```python
from build123d import *

# Parameters (mm, degrees)
EXTRUSION1_DEPTH = 3


with BuildPart() as part:
    # Esquisse1 → Extrusion1 (new body)
    with BuildSketch(Plane.XY):
        with BuildLine():
            Line((150, 232), (-150, 232))
            Line((-150, 232), (-150, 30))
            ThreePointArc((-150, 30), (-135.857864376, 24.142135624), (-130, 10))
            Line((-130, 10), (-130, 0))
            Line((-130, 0), (130, 0))
            Line((130, 0), (130, 10))
            ThreePointArc((130, 10), (135.857864376, 24.142135624), (150, 30))
            Line((150, 30), (150, 232))
        make_face()
        with BuildLine():
            Line((-15, 102), (-15, 132))
            ThreePointArc((-15, 132), (0, 147), (15, 132))
            Line((15, 132), (15, 102))
            ThreePointArc((15, 102), (0, 87), (-15, 102))
        make_face(mode=Mode.SUBTRACT)
        with BuildLine():
            Line((-110, 207), (-110, 217))
            ThreePointArc((-110, 217), (-100, 227), (-90, 217))
            Line((-90, 217), (-90, 207))
            ThreePointArc((-90, 207), (-100, 197), (-110, 207))
        make_face(mode=Mode.SUBTRACT)
    extrude(amount=EXTRUSION1_DEPTH)


solid = part.part
```
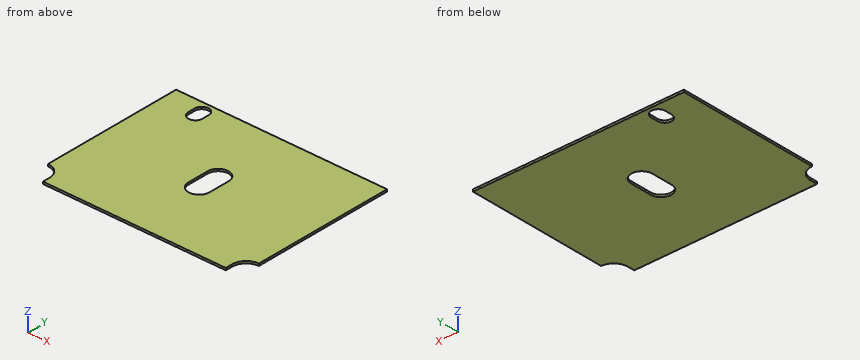
Can you work these out from the model? Positions are in its coordinate system, mm. Give positions to 0.01 mm unless a question says otherwise; leave off trailing zeros. Write each loop counter-clockwise with the first axis right and the second up, starting at its lowest first coordinate (ties: lowest second). Pieces come first, ordered by that corner, then holes. Notation, with made-up numbers: (42.25, 38) -> (96.25, 38) arc R10 ccw to (96.25, 56) -> close; hole circle Ø6 at (-25.5, 35.25). An arc over 180 degrees is marked (long way). One line per item, written item: value.
Q1. Please list where these lines run through material, in increasing order: line 1 (X direction, y = 104, z = 1.7); line 2 (X direction, y = 209, z = 2); line 3 (Y direction, x = 134, z = 0.45). Write a range as [from, to].
Results found:
line 1: x = [-150, -15], [15, 150]
line 2: x = [-150, -110], [-90, 150]
line 3: y = [22, 232]
Q2. Imagine slicing it at B-B on x = -100. Please give me the cut outline in (y, z), and give its area (3 significant figures).
Results found:
outline: (0, 0) -> (197, 0) -> (197, 3) -> (0, 3) -> close; (227, 0) -> (232, 0) -> (232, 3) -> (227, 3) -> close
area: 606 mm^2
Q3. Imagine slicing it at A-A on y = 113.5. Please give me the cut outline in (x, z), and give its area (3 significant figures).
Results found:
outline: (-150, 0) -> (-15, 0) -> (-15, 3) -> (-150, 3) -> close; (15, 0) -> (150, 0) -> (150, 3) -> (15, 3) -> close
area: 810 mm^2
Q4. Imagine slicing it at C-C on z = 2.2. Please give me the cut outline in (x, y), and give its area (3 significant figures).
Results found:
outline: (-150, 30) arc R20 cw to (-130, 10) -> (-130, 0) -> (130, 0) -> (130, 10) arc R20 cw to (150, 30) -> (150, 232) -> (-150, 232) -> close; hole (-110, 207) arc R10 ccw to (-90, 207) -> (-90, 217) arc R10 ccw to (-110, 217) -> close; hole (-15, 102) arc R15 ccw to (15, 102) -> (15, 132) arc R15 ccw to (-15, 132) -> close
area: 66,500 mm^2
